Autodesk Inventor part; units mm, degrees
ref_plane "Start plane" through (0, 0, 0) normal (0, 0, 1) x (1, 0, 0)
ref_plane "End plane" through (0, 0, 1555) normal (0, 0, 1) x (1, 0, 0)
ref_plane "Work Plane4" through (-55, 0, -55) normal (0.7071, 0, -0.7071) x (-0.7071, 0, -0.7071)
ref_plane "Start plane" through (0, 0, 0) normal (0, 0, 1) x (1, 0, 0)
ref_plane "End plane" through (0, 0, 1555) normal (0, 0, 1) x (1, 0, 0)
sketch "Sketch2" plane through (0, 0, 0) normal (0, 0, 1) x (1, 0, 0)
  line L0 (-55, 100.8) -> (-14.95, 100.8)
  line L1 (-55, 110) -> (-55, 100.8)
  line L2 (55, 110) -> (-55, 110)
  line L3 (55, 100.8) -> (55, 110)
  line L4 (14.95, 100.8) -> (55, 100.8)
  line L5 (2.95, -88.8) -> (2.95, 88.8)
  line L6 (55, -100.8) -> (14.95, -100.8)
  line L7 (55, -110) -> (55, -100.8)
  line L8 (-55, -100.8) -> (-55, -110)
  line L9 (-14.95, -100.8) -> (-55, -100.8)
  line L10 (-2.95, 88.8) -> (-2.95, -88.8)
  line L11 (0, -154) -> (0, 154) construction
  line L12 (-2.95, -100.8) -> (2.95, -100.8) construction
  arc A0 (-14.95, -100.8) -> (-2.95, -88.8) centre (-14.95, -88.8) ccw
  arc A1 (-2.95, 88.8) -> (-14.95, 100.8) centre (-14.95, 88.8) ccw
  arc A2 (14.95, 100.8) -> (2.95, 88.8) centre (14.95, 88.8) ccw
  arc A3 (2.95, -88.8) -> (14.95, -100.8) centre (14.95, -88.8) ccw
  line L13 (-77, 0) -> (77, 0) construction
  line L14 (-55, -110) -> (55, -110)
  point P0 (-2.95, 100.8)
  point P1 (2.95, 100.8)
  point P2 (0, 0)
  point P3 (0, -100.8)
  point P4 (0, 0)
  dimension "d1" = 220
  dimension "d3" = 9.2
  dimension "d5" = 5.9
  dimension "d7" = 110
  dimension "d13" = 12
  dimension "d14" = 110
  dimension "d15" = 55
extrude "Body" add sketch "Sketch2" along normal up to surface (1555 mm away) from surface at 0
sketch "Sketch3" plane through (0, 0, 0) normal (0, 0, 1) x (1, 0, 0)
  line L0 (0, 0) -> (10, 0)
ref_plane "Work Plane3" through (0, 0, 0) normal (0, -1, 0) x (1, 0, 0)
ref_plane "Work Plane4" through (-55, 0, -55) normal (0.7071, 0, -0.7071) x (-0.7071, 0, -0.7071)
split "Split1" plane through (-55, 0, -55) removes the side toward (0.7071, 0, -0.7071)
ref_plane "Work Plane5" through (55, 0, -55) normal (-0.7071, 0, -0.7071) x (-0.7071, 0, 0.7071)
split "Split2" plane through (55, 0, -55) removes the side toward (-0.7071, 0, -0.7071)
ref_plane "Work Plane6" through (55, 0, 1555) normal (-0.7071, 0, 0.7071) x (0.7071, 0, 0.7071)
split "Split3" plane through (55, 0, 1555) removes the side toward (-0.7071, 0, 0.7071)
sketch "Sketch4" plane through (0, 0, 0) normal (0, -1, 0) x (1, 0, 0)
  line L0 (-2, 0) -> (12, 0)
  line L1 (-2, 1555) -> (12, 1555)
  dimension "d19" = 1555
equation "\"d1\" = ParH"
equation "\"d3\" = t2"
equation "\"d7\" = b"
equation "\"d13\" = R1"
equation "\"d14\" = 0.5 * d1"
equation "\"d15\" = 0.5 * d7"
equation "\"d8\" = G_L"
equation "\"b\" = 110"
equation "\"ParH\" = 220"
equation "\"R1\" = 12"
equation "\"G_L\" = d19"
equation "\"t1\" = 5.9"
equation "\"t2\" = 9.2"
equation "\"G_OFFSET_START\" = 0"
equation "\"G_OFFSET_END\" = 55"
equation "\"d17\" = G_OFFSET_END + B_L"
properties part number "DIN 1025 - IPE 220-1555" material "Steel, Mild"
Source: CAD feature listing. Evaluate the final solid. Frame: model axes, mm. A direction names the side the tool comes from. Give positions to 0.01 mm unless a question says otherwise; leave off trailing zeros. Write each loop counter-clockwise with the first axis right and the second up, starting at its lowest first coordinate (ties: lowest second). Pieces come first, ordered by that corner, then holes.
1. Section query B-B (z = 875). Return the cut outline in (x, y), then the cut area to 3 significant figures.
2. Section query A-A (y = 16.5). Return the cut outline in (x, z), then the cut area to 3 significant figures.
3. Access query for faces 1 (the face through (-35, 100.8, 740)), 2 (the face through (-1, 1, 1)), 3 (the face through (2.95, -1, 742)). Directions: +Z, -Z, +X, -X, +Y, -Y. A direction counts if a zero-diameter tool reaches every point of the face in a straight line with its end or side. Return the directions, or none.
4. Pull-direction query (Y, two-part tool) for faces 4 (the face through (0, -1, 1500)), 5 (the face through (-35, -100.8, 740)), 6 (the face through (-2.95, 1, 740)), 7 (the face through (1, 110, 767)); classes: +Y half, -Y half, draft (parallel to the pull), parting line (faces both ways), or undercut.
5. First-contact query: pin 1 (1 mm diameter, centred on y = 7, z = 741.5, fed in from -X). Flat tip, straight axial feed; report the tip coordinate or a pass-through.
6. Material intervals for line 1 along Y through (x, z) = (-39, 474); line 2 along X through (y, z) = (47, 82); line 3 along Y through (x, z) = (12.5, 1208.5), sorted ascending.
Output values:
1. outline: (-55, -110) - (55, -110) - (55, -100.8) - (14.95, -100.8) arc R12 cw to (2.95, -88.8) - (2.95, 88.8) arc R12 cw to (14.95, 100.8) - (55, 100.8) - (55, 110) - (-55, 110) - (-55, 100.8) - (-14.95, 100.8) arc R12 cw to (-2.95, 88.8) - (-2.95, -88.8) arc R12 cw to (-14.95, -100.8) - (-55, -100.8) - close
1. area: 3,340 mm2
2. outline: (-2.95, 2.95) - (0, 0) - (2.95, 2.95) - (2.95, 1502.95) - (-2.95, 1497.05) - close
2. area: 8,840 mm2
3. face 1: +Z, -Z, -X
3. face 2: -Z, -X, +Y, -Y
3. face 3: +Z, -Z, +X
4. face 4: draft
4. face 5: undercut
4. face 6: undercut
4. face 7: +Y half
5. pin 1: stops at x = -2.95
6. line 1: y = -110 to -100.8, 100.8 to 110
6. line 2: x = -2.95 to 2.95
6. line 3: y = -110 to -100.55, 100.55 to 110
